The listing builds one solid part. Answer for the finished solid, in the listing's coordinates (mm). Face numbers are marked on the shaded views. A direction names the side the tool comes from. Coordinates: 2 decimals unless noted, no trailing zeros. Order: outer loops, then holes, each group sorted by start corner. A loop starts at its lowest first (then second) coordinate and runs counter-clockwise, first axis right, second up. Notation, with made-up numbers: (-30, 67.5) -> (4, 67.5) arc R15 cw to (4, 96.5) -> close; hole circle Ø3 at (64, 19.25). An arc over 180 degrees is marked (long way). Return JSON: item names as keys, results as strings.
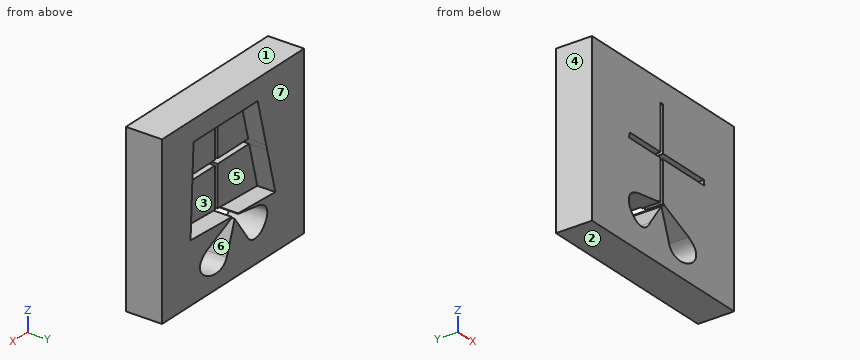
```python
from build123d import *

# Parameters (mm, degrees)
SKETCH1_W           = 16
SKETCH1_H           = 14
BOSS_EXTRUDE1_DEPTH = 3
CUT_EXTRUDE5_DEPTH  = 3
CUT_EXTRUDE6_DEPTH  = 1.5


with BuildPart() as part:
    # Sketch1 → Boss-Extrude1 (new body)
    with BuildSketch(Plane(origin=(0, 0, 0), x_dir=(1, 0, 0), z_dir=(0, 1, 0))):
        with Locations((-34.802547771, 15.318471338)):
            Rectangle(SKETCH1_W, SKETCH1_H)
    extrude(amount=BOSS_EXTRUDE1_DEPTH)

    # Sketch2 → Cut-Extrude5 (cut)
    with BuildSketch(Plane(origin=(0, 3, 0), x_dir=(1, 0, 0), z_dir=(0, 1, 0))):
        with BuildLine():
            Line((-35.361772538, 17.654157516), (-35.361772538, 17.610701513))
            Line((-35.361772538, 17.610701513), (-35.087707093, 17.598006383))
            Line((-35.087707093, 17.598006383), (-35.087707093, 14.224865562))
            Line((-35.087707093, 14.224865562), (-38.648703672, 14.224865562))
            Line((-38.648703672, 14.224865562), (-38.539082436, 13.797679772))
            Line((-38.539082436, 13.797679772), (-35.088327204, 13.797679772))
            Line((-35.088327204, 13.797679772), (-35.088327204, 10.043136726))
            Line((-35.088327204, 10.043136726), (-34.789528654, 10.043136726))
            Line((-34.789528654, 10.043136726), (-34.789528654, 13.797679772))
            Line((-34.789528654, 13.797679772), (-30.176657964, 13.797679772))
            Line((-30.176657964, 13.797679772), (-30.156870066, 14.224865562))
            Line((-30.156870066, 14.224865562), (-34.789528654, 14.224865562))
            Line((-34.789528654, 14.224865562), (-34.789528654, 17.584194303))
            Line((-34.789528654, 17.584194303), (-34.658050894, 17.578104053))
            Line((-34.658050894, 17.578104053), (-34.658050894, 17.654157516))
            Line((-34.658050894, 17.654157516), (-31.911401586, 18.883435151))
            add(Edge.make_bspline(
                [(-31.911401586, 18.883435151), (-29.374274196, 20.248494332), (-33.305897718, 22.135276734), (-34.090701751, 20.417941358)],
                knots=[0, 0, 0, 0, 1, 1, 1, 1], degree=3))
            Line((-34.090701751, 20.417941358), (-34.991899262, 17.868989737))
            Line((-34.991899262, 17.868989737), (-36.257619528, 19.650233345))
            add(Edge.make_bspline(
                [(-36.257619528, 19.650233345), (-37.304461787, 21.759932149), (-40.155684718, 18.540444353), (-37.66921168, 18.003375835)],
                knots=[0, 0, 0, 0, 1, 1, 1, 1], degree=3))
            Line((-37.66921168, 18.003375835), (-35.361772538, 17.654157516))
        make_face()
    extrude(amount=-CUT_EXTRUDE5_DEPTH, mode=Mode.SUBTRACT)

    # Sketch3 → Cut-Extrude6 (cut)
    with BuildSketch(Plane(origin=(0, 3, 0), x_dir=(1, 0, 0), z_dir=(0, 1, 0))):
        Polygon((-35.087707093, 17.598006383), (-39.567544365, 17.805519282), (-37.575619559, 10.043136726), (-30.350574127, 10.043136726), (-30.011512943, 17.362869325), align=None)
    extrude(amount=-CUT_EXTRUDE6_DEPTH, mode=Mode.SUBTRACT)


solid = part.part
```
Item 1: Determine the mould class of the marked faces 1, 2, 3 and 4 for opening direction Z: pulls with the +Z half, pulls with the -Z half, needs draft (parallel to the pull), parting line crosses it, or undercut.
Answer list:
{"face 1": "pulls with the +Z half", "face 2": "pulls with the -Z half", "face 3": "undercut", "face 4": "needs draft"}
Item 2: The part is cut by section D-D on z = -14. Determine the outline of the cut face in (x, y), plus the area to 3 significant figures.
Answer list:
{"outline": "(-42.8, 0) -> (-38.59, 0) -> (-38.59, 3) -> (-42.8, 3) -> close; (-30.17, 0) -> (-26.8, 0) -> (-26.8, 3) -> (-30.17, 3) -> close", "area": "22.7 mm2"}
Item 3: A flat-ended cylindrical pin translates along its axis: pin 1 (1 mm diameter, centred on x = -37.5, z = -12, fed in from +Y). Find the tip coordinate at first contact, or state that the pin passes through.
Answer list:
{"pin 1": "y = 1.5"}
Item 4: Which of the six approach directions +Z, -Z, +X, -X, +Y, -Y give full straight-line access (tool end or side, diameter ignored) to the marked faces 5, 6 and 7?
Answer list:
{"face 5": "+Y", "face 6": "+Y, -Y", "face 7": "+Z, -Z, +X, -X, +Y"}
Item 5: Find the intervals of material crossed by probe 1 along Z at (x, y) = (-30.75, 0.15); probe 2 along X at (y, z) = (1.6, -19.5); probe 3 along Z at (x, y) = (-31.75, 0.65), in increasing order.
Answer list:
{"probe 1": "-22.32 to -14.22, -13.8 to -8.32", "probe 2": "-42.8 to -38.51, -36.15 to -34.42, -31.18 to -26.8", "probe 3": "-22.32 to -20.8, -18.98 to -14.22, -13.8 to -8.32"}
Item 6: The part is cut by section B-B on x = -36. Determine the outline of the cut face in (y, z), plus the area to 3 significant figures.
Answer list:
{"outline": "(0, -22.32) -> (3, -22.32) -> (3, -19.29) -> (0, -19.29) -> close; (0, -17.75) -> (3, -17.75) -> (3, -17.64) -> (1.5, -17.64) -> (1.5, -14.22) -> (0, -14.22) -> close; (0, -13.8) -> (1.5, -13.8) -> (1.5, -10.04) -> (3, -10.04) -> (3, -8.32) -> (0, -8.32) -> close", "area": "25.4 mm2"}
Item 7: The part is cut by section C-C on z = -18.5. Count the separate pieces of the cut face and the enclosed holes in it, plus the area to 3 significant figures.
Answer list:
{"separate pieces": "3", "enclosed holes": "0", "area": "32.7 mm2"}
Item 8: The part is cut by section A-A on z = -15.75. Determine the outline of the cut face in (x, y), plus the area to 3 significant figures.
Answer list:
{"outline": "(-42.8, 0) -> (-35.09, 0) -> (-35.09, 1.5) -> (-39.04, 1.5) -> (-39.04, 3) -> (-42.8, 3) -> close; (-34.79, 0) -> (-26.8, 0) -> (-26.8, 3) -> (-30.09, 3) -> (-30.09, 1.5) -> (-34.79, 1.5) -> close", "area": "34.1 mm2"}
